Autodesk Inventor part; units mm, degrees
ref_plane "YZ Plane" through (0, 0, 0) normal (1, 0, 0) x (0, 1, 0)
ref_plane "XZ Plane" through (0, 0, 0) normal (0, 1, 0) x (-1, 0, 0)
ref_plane "XY Plane" through (0, 0, 0) normal (0, 0, 1) x (1, 0, 0)
sketch "Sketch1" plane through (0, 0, 0) normal (0, 1, 0) x (-1, 0, 0)
  circle A0 centre (0, 0) radius 13.4938
  dimension "d0" = 26.9875
extrude "Extrusion1" add sketch "Sketch1" along normal blind 38.1
sketch "Sketch2" plane through (0, 38.1, 0) normal (0, 1, 0) x (1, 0, 0)
  circle A0 centre (0, 0) radius 5.1594
  dimension "d3" = 10.3187
extrude "Extrusion2" add sketch "Sketch2" along normal blind 3.175
sketch "Sketch3" plane through (0, 38.1, 0) normal (0, 1, 0) x (1, 0, 0)
  circle A0 centre (-7.9375, 0) radius 1.524
  line L0 (0, 0) -> (-7.9375, 0) construction
  line L1 (0, -15.84) -> (0, 17.6643) construction
  circle A1 centre (7.9375, 0) radius 1.524
  line L2 (0, 0) -> (7.9375, 0) construction
  dimension "d6" = 3.048
  dimension "d7" = 7.9375
  dimension "d8" = 0
  dimension "d9" = 17.6643
  dimension "d10" = 15.8399
extrude "Extrusion3" cut sketch "Sketch3" against normal blind 3.175
sketch "Sketch6" plane through (0, 41.275, 0) normal (0, 1, 0) x (1, 0, 0)
  circle A0 centre (0, 0) radius 1.1557
  dimension "d18" = 2.3114
extrude "Extrusion6" add sketch "Sketch6" along normal blind 19.05
properties part number "motor"
Model file for the job. Use its own axes, mm. A direction names the side the tool comes from. Coordinates: 2 decimals unless noted, no trailing zeros. Loops run counter-clockwise (first coordinate to the right, second up) from the corner with the lowest first, then second, coordinate; pieces in that order, holes last. Notation, with made-up numbers: (31, 34.5) - (37, 34.5) arc R27 cw to (37, 63.5) - close; hole circle Ø2 at (-13.75, 37.25). An arc over 180 degrees is marked (long way). Answer as a JSON object with one key per item and string values. Group by question number.
(1) Tool access for faces 1 (the face through (0, 0, 0)), 2 (the face through (-6, 38.1, 0)): list every direction of +Z, -Z, +X, -X, +Y, -Y with a clear straight run to the whole face (end or side of a thin tool).
(2) Probe line 1 along Y through (x, z) = (-11, 7.25); line 2 along X through (y, z) = (44, 0); line 3 along Y through (x, z) = (-9, 1) (3 decimals). List the from-to ranges inside material, lowest first.
(3) Cut at A-A (x = 0). Give the cut face in (y, z) (3 decimals), then the cut area to 3 significant figures.
(4) Cut at C-C (y = 49.5). Give the cut face in (x, z).
(5) Two-plate mould, pull along X, no slides. Class faces 3 (the face through (8, 34.925, 0)), 4 (the face through (-8, 34.925, 0)), 5 (the face through (0, 60.325, 0)), 6 (the face through (-12.87, 18.78, -4.05)): released by +X, released by -X, zero draft, split by the parting line, or undercut.
(6) Flat gauge pins, fed straight in: pin 1 (2 mm diameter, centred on x = -4.5, y = 30.5, fed in from -Z); pin 2 (1.8 mm diameter, centred on x = -7.94, z = 0, fed in from +Y) (3 decimals); pin 3 (1.5 mm diameter, centred on y = 28.5, z = -9, fed in from -X). Where does each tip first touch, or does it go through?
(7) Cut at D-D (y = 36.5). Give the cut face in (x, z).
(8) Cut at B-B (z = 0). Give the cut face in (x, y) (1 decimal), then the cut area to 3 significant figures.
Geometry says:
{
 "1": {"face 1": "+Z, -Z, +X, -X, -Y", "face 2": "+Y"},
 "2": {"line 1": "y = 0 to 38.1", "line 2": "x = -1.16 to 1.16", "line 3": "y = 0 to 34.925"},
 "3": {"outline": "(0, -13.494) - (38.1, -13.494) - (38.1, -5.159) - (41.275, -5.159) - (41.275, -1.156) - (60.325, -1.156) - (60.325, 1.156) - (41.275, 1.156) - (41.275, 5.159) - (38.1, 5.159) - (38.1, 13.494) - (0, 13.494) - close", "area": "1,110 mm^2"},
 "4": {"outline": "circle Ø2.31 at (0, 0)"},
 "5": {"face 3": "undercut", "face 4": "undercut", "face 5": "zero draft", "face 6": "split by the parting line"},
 "6": {"pin 1": "stops at z = -13.03", "pin 2": "stops at y = 34.925", "pin 3": "stops at x = -10.68"},
 "7": {"outline": "circle Ø26.99 at (0, 0); hole circle Ø3.05 at (-7.94, 0); hole circle Ø3.05 at (7.94, 0)"},
 "8": {"outline": "(-13.5, 0) - (13.5, 0) - (13.5, 38.1) - (9.5, 38.1) - (9.5, 34.9) - (6.4, 34.9) - (6.4, 38.1) - (5.2, 38.1) - (5.2, 41.3) - (1.2, 41.3) - (1.2, 60.3) - (-1.2, 60.3) - (-1.2, 41.3) - (-5.2, 41.3) - (-5.2, 38.1) - (-6.4, 38.1) - (-6.4, 34.9) - (-9.5, 34.9) - (-9.5, 38.1) - (-13.5, 38.1) - close", "area": "1,090 mm^2"}
}
